Study the drawing (mm; zero at the part's minimum x, y, z) and answer. A direction names the side the tool comes from. Give positions to 0.01 mm unless a question says otherwise; leave off trailing zeros. Order: outer loops, then holes, each group sorted by start corner. A loop starts at its lowest first (then second) coordinate and runs counter-clockwise, first axis right, second up. Notation, with made-up numbers: (34, -12) - (53, -12) arc R33 ccw to (53, 17) - close; hole circle Ø9 at (86, 76). An arc over 180 degrees is marked (long way). Return JSON: item names as keys, results as strings.
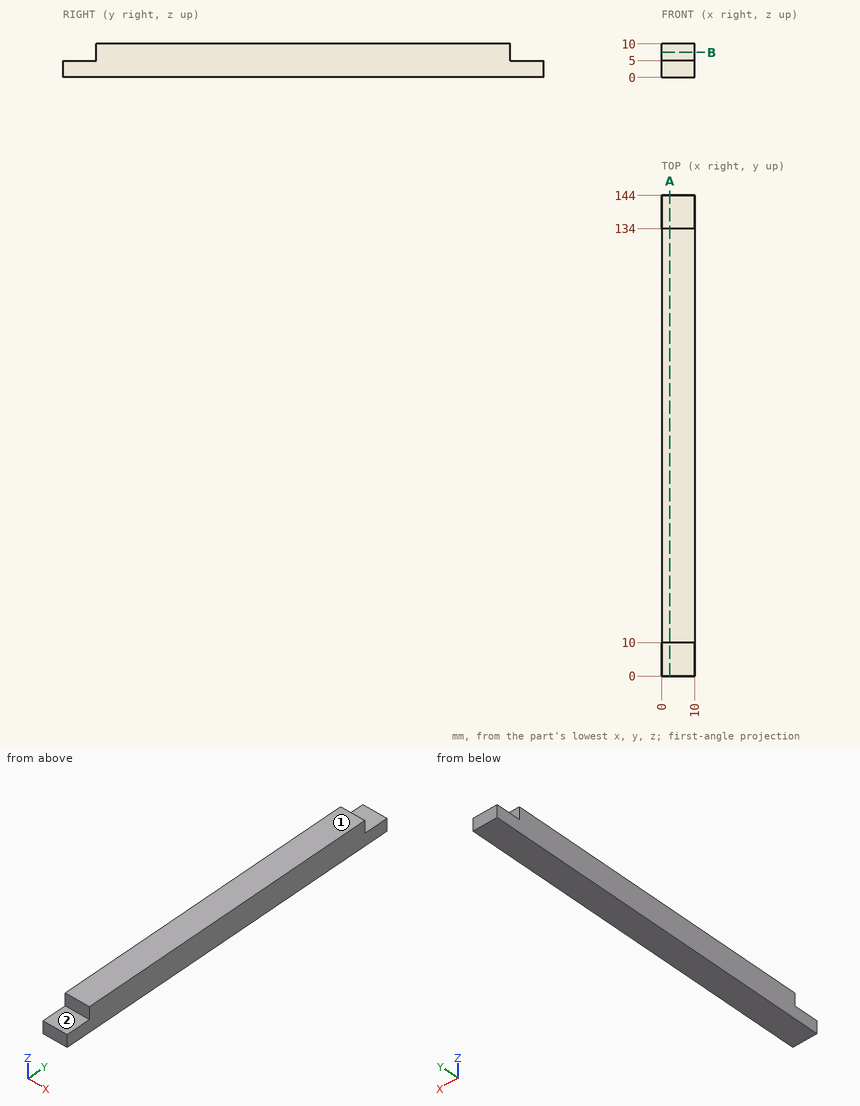
Q1. Given pin 1 (3 mm diameter, centred on x = 4, y = 141, fed in from +Z); pin 2 (4 mm diameter, centred on x = 3, z = 7.5, fed in from +Y), each flat-ended and moving along its own axis, determine where each tip first touches the part or whether it passes through.
Values:
{"pin 1": "stops at z = 5", "pin 2": "stops at y = 134"}
Q2. A cutting plane is placed at A-A (x = 2.5). Write down the section's boundary in (y, z).
Values:
{"outline": "(0, 0) - (144, 0) - (144, 5) - (134, 5) - (134, 10) - (10, 10) - (10, 5) - (0, 5) - close"}
Q3. For the marked faces 1 and 2, determine the directions among +Z, -Z, +X, -X, +Y, -Y from which every point of the face is accessible in a straight line to the end or side of a thin tool.
Values:
{"face 1": "+Z, +X, -X, +Y, -Y", "face 2": "+Z, +X, -X, -Y"}
Q4. Consider L1, parallel to Y at x = 4, z = 7.25. Determine where the line is inside the solid, lowest interval first.
Values:
{"L1": "y = 10 to 134"}
Q5. A cutting plane is placed at B-B (z = 7.5). Write down the section's boundary in (x, y).
Values:
{"outline": "(0, 10) - (10, 10) - (10, 134) - (0, 134) - close"}
